Autodesk Inventor part; units mm, degrees
ref_plane "YZ Plane" through (0, 0, 0) normal (1, 0, 0) x (0, 1, 0)
ref_plane "XZ Plane" through (0, 0, 0) normal (0, 1, 0) x (-1, 0, 0)
ref_plane "XY Plane" through (0, 0, 0) normal (0, 0, 1) x (1, 0, 0)
sketch "Sketch1" plane through (0, 0, 0) normal (0, 0, 1) x (1, 0, 0)
  line L0 (-61.5, -83.5) -> (62.5, -83.5)
  line L1 (62.5, -83.5) -> (62.5, 73.5)
  line L2 (62.5, 73.5) -> (-61.5, 73.5)
  line L3 (-61.5, 73.5) -> (-61.5, -83.5)
  line L4 (-67.5, -94.5) -> (67.5, -94.5)
  line L5 (67.5, -94.5) -> (67.5, 91.5)
  line L6 (62.5, -70.5) -> (-20.5, -70.5)
  line L7 (-20.5, 73.5) -> (62.5, 73.5)
  line L8 (62.5, 73.5) -> (62.5, -70.5)
  line L9 (67.5, 91.5) -> (-67.5, 91.5)
  line L10 (-67.5, 91.5) -> (-67.5, -94.5)
  circle A0 centre (61.2932, 86.5) radius 2
  circle A1 centre (61.2932, -89.3536) radius 2
  circle A2 centre (-62.5, -89.3536) radius 2
  circle A3 centre (-62.5, 86.5) radius 2
  line L11 (-64.5, -83.5) -> (-64.5, 80.5)
  line L12 (-58.5, 86.5) -> (-64.5, 80.5)
  line L13 (-58.5, 86.5) -> (-30.5, 86.5)
  line L14 (-30.5, 86.5) -> (-30.5, 24)
  line L15 (-30.5, 24) -> (-20.5, 24)
  line L16 (-20.5, 24) -> (-20.5, 73.5)
  line L17 (-20.5, -70.5) -> (-20.5, -21)
  line L18 (-20.5, -21) -> (-30.5, -21)
  line L19 (-30.5, -21) -> (-30.5, -89.5)
  line L20 (-30.5, -89.5) -> (-58.5, -89.5)
  line L21 (-64.5, -83.5) -> (-58.5, -89.5)
  point P0 (0, 0)
  point P1 (67.5, -91)
  point P2 (67, 91.5)
  point P3 (-67, 91.5)
  point P4 (-67.5, 91)
extrude "Extrusion1" add sketch "Sketch1" along normal blind 35 contours L3 L2 L14 L15 L16 L1 L6 L17 L18 L19 L0 | L0 L19 L20 L21 L11 L12 L13 L14 L2 L3 | L19 L18 L17 L6 L1 L0 | L2 L16 L15 L14 | L10 L9 L5 L4 | A0 | A1 | A2 | A3
sketch "Skizze3" plane through (0, 0, 35) normal (0, 0, 1) x (1, 0, 0)
  circle A0 centre (61.2932, 86.5) radius 2
  circle A1 centre (-62.5, 86.5) radius 2
  circle A2 centre (61.2932, -89.3536) radius 2
  circle A3 centre (-62.5, -89.3536) radius 2
  point P0 (0, 0)
hole "Bohrung1" at (-62.5, 86.5, 35) at (61.2932, 86.5, 35) at (61.2932, -89.3536, 35) at (-62.5, -89.3536, 35) direction (0, 0, -1) diameter 3.4 end through all counterbore diameter 6.5 counterbore depth 3.4
sketch "Skizze4" plane through (0, 0, 0) normal (0, 0, -1) x (-1, 0, 0)
  line L0 (-57.5, 84.5) -> (57.5, 84.5)
  line L1 (57.5, 84.5) -> (57.5, -84.5)
  line L2 (57.5, -84.5) -> (-57.5, -84.5)
  line L3 (-57.5, -84.5) -> (-57.5, 84.5)
  line L4 (-57.5, 84.5) -> (57.5, -84.5) construction
  line L5 (57.5, 84.5) -> (-57.5, -84.5) construction
  line L6 (67.5, 91.5) -> (67.5, -94.5)
  line L7 (67.5, -94.5) -> (-67.5, -94.5)
  point P0 (0, 0)
  dimension "d14" = 10
  dimension "d15" = 10
extrude "Extrusion3" cut sketch "Skizze4" against normal blind 30
chamfer "Fasen2" distance 1 angle 45 4 edges at (-67.5, -94.5, 17.5) (-67.5, 91.5, 17.5) (67.5, 91.5, 17.5) (67.5, -94.5, 17.5)
chamfer "Fasen3" distance 1 angle 45 8 edges at (-67.5, -1.5, 35) (0, 91.5, 35) (67.5, -1.5, 35) (0, -94.5, 35) (-67, -94, 35) (67, -94, 35) (67, 91, 35) (-67, 91, 35)
properties part number "Kameraturm_Deckel"
For this review, take the finished solid that the model builds, in its own axes (mm). A direction names the side the tool comes from. Round coordinates to 2 decimals unless told otherwise and drop trailing zeros. Order: outer loops, then holes, each group sorted by start corner. A loop starts at its lowest first (then second) coordinate and runs counter-clockwise, first axis right, second up.
Q1. We need section A-A, the plane y = 15. Give the boundary of the cut face in (x, z), plus the area to 3 significant figures.
Findings below:
outline: (-67.5, 0) - (-57.5, 0) - (-57.5, 30) - (57.5, 30) - (57.5, 0) - (67.5, 0) - (67.5, 34) - (66.5, 35) - (-66.5, 35) - (-67.5, 34) - close
area: 1,270 mm2
Q2. Wall thickness on line 1 (X direction, y = 86.5, z = 11); line 2 (Y direction, x = -62.5, z = 33.8); line 3 (Y direction, x = 14, z = 14): over which ranges is each line inside the solid? List them lowest first.
Findings below:
line 1: x = -67.5 to -64.2, -60.8 to 59.59, 62.99 to 67.5
line 2: y = -94.5 to -92.6, -86.1 to 83.25, 89.75 to 91.5
line 3: y = -94.5 to -84.5, 84.5 to 91.5
Q3. Insertion check: P1, Ø12, axis at x = -42.5, y = 16, coming from the -Z side; P2, Ø2, axis at x = -61, y = 85.5, coming from the +Z side. Each pin has a flat end and moves straight along its axis. Give the tip position at first contact, or say it passes through.
Findings below:
P1: stops at z = 30
P2: stops at z = 31.6
Q4. We need section C-C, the plane z = 16.5. Give the boundary of the cut face in (x, y).
Findings below:
outline: (-67.5, -93.5) - (-66.5, -94.5) - (66.5, -94.5) - (67.5, -93.5) - (67.5, 90.5) - (66.5, 91.5) - (-66.5, 91.5) - (-67.5, 90.5) - close; hole circle Ø3.4 at (-62.5, -89.35); hole circle Ø3.4 at (-62.5, 86.5); hole (-57.5, -84.5) - (57.5, -84.5) - (57.5, 84.5) - (-57.5, 84.5) - close; hole circle Ø3.4 at (61.29, -89.35); hole circle Ø3.4 at (61.29, 86.5)
Q5. Mouldability with a two-part tool opening along Y and no side actions: class faces 4 (the flat face through (-57.5, 1, 15)), 5 (the flat face through (-67.5, 0, 17)), 6 (the cylindrical face through (-63.476, -92.454, 33.276)), 7 (the flat face through (1, 91.5, 17)) as pulls with the +Y half, pulls with the -Y half, needs draft (parallel to the pull), parting line crosses it, or undercut.
Findings below:
face 4: undercut
face 5: needs draft
face 6: undercut
face 7: pulls with the +Y half
Q6. Machinability: for faces 1 (the flat face through (-61, 85, 31.6)), 2 (the flat face through (-60, 6, 0)), 3 (the flat face through (-1, -84.5, 15)), which of the approach directions +Z, -Z, +X, -X, +Y, -Y give a long, thin tool a straight path to every point of the face, cutting with its end or side? Answer none if there is none.
Findings below:
face 1: +Z
face 2: -Z, +X, -X, +Y, -Y
face 3: -Z
Q7. We need section B-B, the plane x = -23. Give the boundary of the cut face in (y, z).
Findings below:
outline: (-94.5, 0) - (-84.5, 0) - (-84.5, 30) - (84.5, 30) - (84.5, 0) - (91.5, 0) - (91.5, 34) - (90.5, 35) - (-93.5, 35) - (-94.5, 34) - close
